The model under review builds one solid part; all positions refer to its coordinate system, in mm. A direction names the side the tool comes from. Give positions to 0.01 mm unless a question says otherwise; leave off trailing zeros. Order: outer loops, then holes, each group sorted by start corner. A loop starts at its lowest first (then second) coordinate and runs counter-clockwise, first axis right, second up. Notation, with made-up numbers: (59, 79) - (67, 79) arc R4 ccw to (67, 84) - close; hole circle Ø3 at (-38.75, 20). An arc over 180 degrees is marked (long way). Use a Markdown table: item, result. Add a question column.
```python
from build123d import *

# Parameters (mm, degrees)
F0_W     = 600
F0_H     = 600
F1_DEPTH = 520
F2_R     = 299.99999
F3_W     = 520
F3_H     = 270
F3_W_2   = 500
F3_H_2   = 250
F4_DEPTH = 150
F5_R     = 25
F6_DEPTH = 300


# Not quite as in the source:
# - a fillet or chamfer is up to 0.001 mm smaller than in the source, because OpenCascade refuses the exact size


with BuildPart() as f1:
    # F0 (on Front) → F1 (new body)
    with BuildSketch(Plane.XZ):
        Rectangle(F0_W, F0_H)
    extrude(amount=F1_DEPTH)

    # F2 (radius 300 in the source; OpenCascade refuses exactly that, so slightly less here)
    f2_edges = [f1.edges().sort_by_distance(p)[0] for p in [
        (300, -260, 300),
        (300, -260, -300),
        (-300, -260, -300),
    ]]
    fillet(f2_edges, radius=F2_R)

    # F3 (on face) → F4 (join)
    with BuildSketch(Plane(origin=(-300, 0, 0), x_dir=(0, -1, 0), z_dir=(-1, 0, 0))):
        with Locations((260, 165)):
            Rectangle(F3_W, F3_H)
        with Locations((260, 165)):
            Rectangle(F3_W_2, F3_H_2, mode=Mode.SUBTRACT)
    extrude(amount=F4_DEPTH)

    # F5 (on face) → F6 (cut)
    with BuildSketch(Plane(origin=(0, 0, 0), x_dir=(-1, 0, 0), z_dir=(0, 1, 0))):
        Circle(F5_R)
    extrude(amount=-F6_DEPTH, mode=Mode.SUBTRACT)


solid = f1.part
```
Q1. Wall thickness on probe 1 along X at (y, z) = (-273, -14); probe 2 along X at (y, z) = (-196, 143); probe 3 along X at (y, z) = (-451, 224.5): over which ranges is each line inside the solid? List them lowest first.
Q2. We need section C-C (z = 171). Write out the cut boundary in (x, y), plus the area to 3 significant figures.
Q3. Clearance check with flat-ended pins moving along their axes: P1, Ø6, axis at x = 98, y = -86.5, coming from the +Z side; P2, Ø5, axis at x = -176, y = -292, coming from the -Z side; P3, Ø3, axis at x = -81, y = -455, coming from the -Z side. State where each tip first meets the part, or that it passes through.
Q4. Draft analysis for pull direction Z (two halves, no side actions). For faces 5 (the flat face through (-374, -510, 163)), 6 (the cylindrical face through (214.45, -263.64, 209.79)), 7 (the flat face through (-374, -256, 30)), state which applies: pulls with the +Z half, pulls with the -Z half, needs draft (parallel to the pull), parting line crosses it, or undercut.
Q5. We need section B-B (x = -310). Write out the cut boundary in (y, z), plus the area to 3 significant figures.
Q6. Machinability: for faces 1 (the flat face through (-300, -256, 15)), 2 (the flat face through (0, -300, 0)), 3 (the flat face through (-374, -256, 40)), 4 (the flat face through (-450, -182, 36)), which of the approach directions +Z, -Z, +X, -X, +Y, -Y give a long, thin tool a straight path to every point of the face, cutting with its end or side? Answer none if there is none.
Q7. We need section D-D (x = -191). Write out the cut boundary in (y, z).
Here are the results:
| question | item | result |
|---|---|---|
| 1 | probe 1 | -299.67 to -20.71, 20.71 to 299.67 |
| 1 | probe 2 | -300 to 263.73 |
| 1 | probe 3 | -300 to 199 |
| 2 | outline | (-450, -520) - (246.49, -520) - (246.49, 0) - (-450, 0) - (-450, -10) - (-300, -10) - (-300, -510) - (-450, -510) - close |
| 2 | area | 287,000 mm2 |
| 3 | P1 | z = 284.56 |
| 3 | P2 | z = -244.74 |
| 3 | P3 | z = -289.27 |
| 4 | face 5 | undercut |
| 4 | face 6 | pulls with the +Z half |
| 4 | face 7 | pulls with the -Z half |
| 5 | outline | (-520, 30) - (0, 30) - (0, 300) - (-520, 300) - close; hole (-510, 40) - (-10, 40) - (-10, 290) - (-510, 290) - close |
| 5 | area | 15,400 mm2 |
| 6 | face 1 | -Z, -X, +Y, -Y |
| 6 | face 2 | +Y |
| 6 | face 3 | -X |
| 6 | face 4 | +Z, -Z, -X, +Y, -Y |
| 7 | outline | (-520, -231.34) - (0, -231.34) - (0, 300) - (-520, 300) - close |
